Input: part model. Units: mm. Frame: model coordinates. Face numbers are marked on the shaded views. A direction names the side the tool comes from. Coordinates: 2 decimals unless noted, no trailing zeros. Order: outer loops, then holes, each group sorted by start corner. A loop starts at its lowest first (then second) coordinate and runs counter-clockwise, first axis right, second up.
from build123d import *
from OCP.BRepFilletAPI import BRepFilletAPI_MakeChamfer

# Parameters (mm, degrees)
SKETCH_2_R          = 9
CUT_EXTRUDE_1_DEPTH = 27.570660511
CHAMFER_1_SIZE      = 1
CHAMFER_1_SIZE2     = 2
CHAMFER_2_SIZE      = 1


with BuildPart() as part:
    # 草图1 → 旋转1 (revolve)
    with BuildSketch(Plane.XY, mode=Mode.PRIVATE) as revolve_1_sk:
        Polygon((0, 0), (13, 0), (13, 12), (12, 12), (12, 13), (15, 13), (15, 16), (0, 16), align=None)
    revolve(revolve_1_sk.sketch.rotate(Axis((0, 16, 0), (0, -1, 0)), 90), axis=Axis((0, 16, 0), (0, -1, 0)))

    # 草图2 → 切除-拉伸1 (cut, through all)
    with BuildSketch(Plane(origin=(0, 16, 0), x_dir=(1, 0, 0), z_dir=(0, 1, 0))):
        with Locations(Location((0, 0, 0), (0, 0, 180))):
            Circle(SKETCH_2_R)
    extrude(amount=-CUT_EXTRUDE_1_DEPTH, mode=Mode.SUBTRACT)

    # 倒角1: one chamfer whose edges measure the first distance from different faces: ONE call of the kernel's chamfer builder (chamfer() names one face for all edges)
    chamfer_1_edges_1 = [part.edges().sort_by_distance(p)[0] for p in [
        (0, 16, -15),
    ]]
    chamfer_1_side_1 = [part.faces().sort_by_distance(p)[0] for p in [
        (0, 14.5, -15),
    ]]
    chamfer_1_edges_2 = [part.edges().sort_by_distance(p)[0] for p in [
        (0, 0, -13),
    ]]
    chamfer_1_side_2 = [part.faces().sort_by_distance(p)[0] for p in [
        (0, 0, -12.632304474),
    ]]
    chamfer_1 = BRepFilletAPI_MakeChamfer(part.part.solid().wrapped)
    for e in chamfer_1_edges_1:
        chamfer_1.Add(CHAMFER_1_SIZE, CHAMFER_1_SIZE2, e.wrapped, chamfer_1_side_1[0].wrapped)  # the first distance lies on this face
    for e in chamfer_1_edges_2:
        chamfer_1.Add(CHAMFER_1_SIZE, CHAMFER_1_SIZE2, e.wrapped, chamfer_1_side_2[0].wrapped)  # the first distance lies on this face
    add(Compound.cast(chamfer_1.Shape()), mode=Mode.REPLACE)

    # 倒角2
    chamfer_2_edges = [part.edges().sort_by_distance(p)[0] for p in [
        (9, 0, 0),
        (9, 16, 0),
        (0, 12, -13),
    ]]
    chamfer(chamfer_2_edges, length=CHAMFER_2_SIZE - 0.0001)  # a hair under: the kernel refuses the full size


solid = part.part
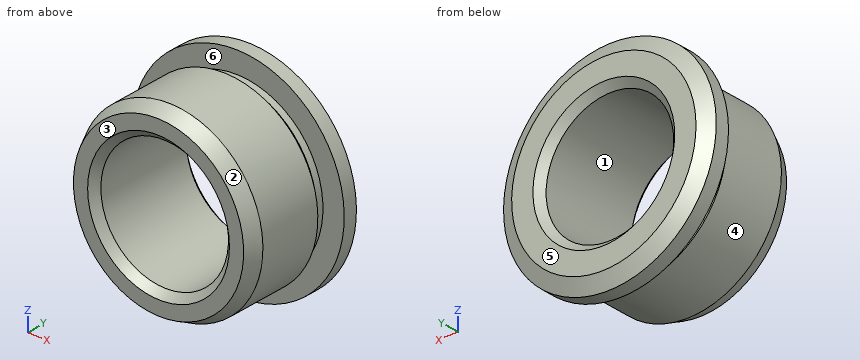
Item 1: Access query for the marked faces 4, 5 and 6. Directions: +Z, -Z, +X, -X, +Y, -Y. A direction counts if a zero-diameter tool reaches every point of the face in a straight line with its end or side. Return the directions, or none.
Response values:
face 4: -Y
face 5: +Z, -Z, +X, -X, +Y
face 6: none
Item 2: Ray query, probe 1 along X at (y, z) = (15.5, 6.5); probe 2 along X at (y, z) = (8.75, 5); probe 3 along Z at (x, y) = (-1, 12.25). Return the intervals inside material, ascending.
Response values:
probe 1: x = -12.4 to -6.93, 6.93 to 12.4
probe 2: x = -12 to -7.48, 7.48 to 12
probe 3: z = -11.96 to -8.94, 8.94 to 11.96
Item 3: Cut plane C-C on y = 6. Return loops of the section in (x, z).
Response values:
outline: circle Ø26 at (0, 0); hole circle Ø18 at (0, 0)
Item 4: Pin query (flat end, axial travel): pin 1 Ø3 at (y, z) = (11, 1) entering from -X; pin 2 Ø3 at (x, y) = (-9, 10) entering from +Z; pin 3 Ø1.5 at (y, z) = (3.5, -2.5) entering from -X. Return the tip coordinate at first contact, or that it passes through.
Response values:
pin 1: stops at x = -13
pin 2: stops at z = 10.62
pin 3: stops at x = -12.88
Item 5: Draft query along Z for the marked faces 1, 2 and 3. Return one class per face: pulls with the +Z half, pulls with the -Z half, needs draft (parallel to the pull), parting line crosses it, or undercut.
Response values:
face 1: undercut
face 2: parting line crosses it
face 3: needs draft
